Verification items for this drawing (mm, ordinates from the low corner). A direction names the side the tool comes from. Round coordinates to 2 decimals unless told otherwise and drop trailing zeros. Order: outer loops, then holes, each group sorted by start corner. A loop starts at its lowest first (then second) coordinate and runs counter-clockwise, first axis right, second up.
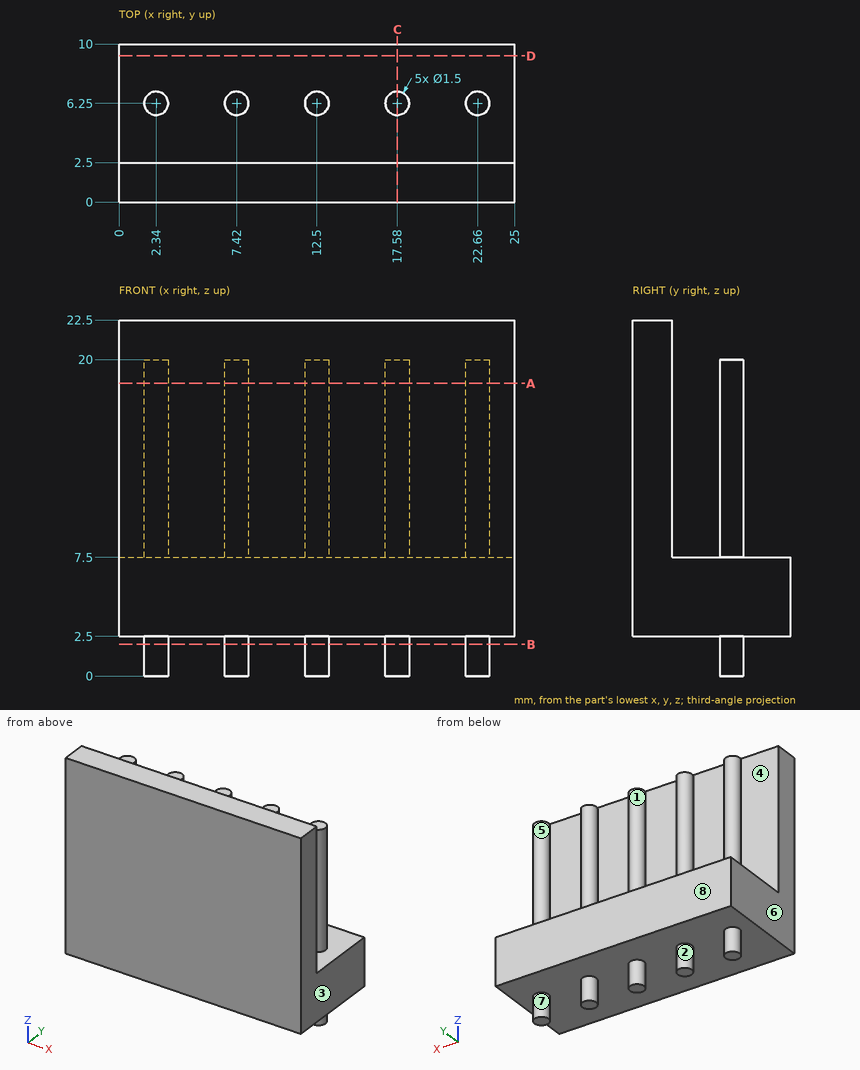
Item 1: Access from +Z, -Z, +X, -X, +Y, -Y to the whole of each face (thin tool, end or side, straight path). Record for the marked faces 4, 5, 6, 7 and 8.
Answer:
face 4: +Z, +X, -X
face 5: +Z
face 6: +Z, -Z, -X, +Y, -Y
face 7: -Z
face 8: +Z, -Z, +X, -X, +Y
Item 2: Release check for a two-part mould opening along Y. For the marked faces 1, 2 and 3 record: released by +Y, released by -Y, zero draft, split by the parting line, or undercut.
Answer:
face 1: undercut
face 2: split by the parting line
face 3: zero draft
Item 3: Scan lines: line 1 along X through (y, z) = (6.75, 12.25); line 2 along Z through (x, y) = (3.5, 5.75); line 3 along Y through (x, z) = (1.5, 12.75). Record each from-to range of solid material in increasing order.
Answer:
line 1: x = 1.78 to 2.9, 6.86 to 7.98, 11.94 to 13.06, 17.02 to 18.14, 22.1 to 23.22
line 2: z = 2.5 to 7.5
line 3: y = 0 to 2.5
Item 4: Sectioned sample at C-C (x = 17.58). Record the cut outline in (y, z), and give its area (3 significant figures).
Answer:
outline: (0, 2.5) - (5.5, 2.5) - (5.5, 0) - (7, 0) - (7, 2.5) - (10, 2.5) - (10, 7.5) - (7, 7.5) - (7, 20) - (5.5, 20) - (5.5, 7.5) - (2.5, 7.5) - (2.5, 22.5) - (0, 22.5) - close
area: 110 mm2
Item 5: Sectioned sample at D-D (y = 9.25). Record the cut outline in (x, z), and give its area (3 significant figures).
Answer:
outline: (0, 2.5) - (25, 2.5) - (25, 7.5) - (0, 7.5) - close
area: 125 mm2
Item 6: Sectioned sample at A-A (z = 18.5). Record the cut outline in (x, y), and give its area (3 significant figures).
Answer:
outline: (0, 0) - (25, 0) - (25, 2.5) - (0, 2.5) - close; circle Ø1.5 at (2.34, 6.25); circle Ø1.5 at (7.42, 6.25); circle Ø1.5 at (12.5, 6.25); circle Ø1.5 at (17.58, 6.25); circle Ø1.5 at (22.66, 6.25)
area: 71.3 mm2
Item 7: Sectioned sample at B-B (z = 2). Record the cut outline in (x, y).
Answer:
outline: circle Ø1.5 at (2.34, 6.25); circle Ø1.5 at (7.42, 6.25); circle Ø1.5 at (12.5, 6.25); circle Ø1.5 at (17.58, 6.25); circle Ø1.5 at (22.66, 6.25)
Item 8: Go/stop test with flat-tipped pins: P1, Ø1.6, axis at x = 17.5, y = 6.5, coming from the +Z side; P2, Ø6, axis at y = 8.5, z = 14.5, coming from the +X side; P3, Ø1.5, axis at x = 13.5, y = 2.5, coming from the -Z side. Record where each tip stops, or that it passes through.
Answer:
P1: stops at z = 20
P2: stops at x = 23.41
P3: stops at z = 2.5
